Build history of the part. All positions in model axes, mm. Give positions to 0.01 mm unless a question says otherwise; leave off trailing zeros. Loops run counter-clockwise (first coordinate to the right, second up) from the corner with the lowest first, then second, coordinate; pieces in that order, holes last.
1) Wall check: line 1 (Z direction, x = 0, y = -228); line 2 (Y direction, x = 0.05, z = 16); line 3 (Z direction, x = 0.1, y = -166). Give the ranges that are in metal, low to high.
2) Band-saw the part on A-A on x = 0. List the corners of the cut face in (y, z).
3) Band-saw the part on B-B on y = -173. List the corners of the cut face in (x, z).
4) Flat gauge pin, fed straight in: P1, Ø6, axis at y = -182.5, z = 6.5, coming from the -X side. Where does the tip first touch, or does it go through?
```python
from build123d import *

# Parameters (mm, degrees)
NATIVE_HOLLOW_UTILITY_SWEEP_PROFILE_R = 0.18


with BuildPart() as part:
    # Native hollow utility sweep: sweep along a path in Illustrative smooth utility route
    with BuildLine(Plane(origin=(0, 0, 0), x_dir=(0, 0, -1), z_dir=(1, 0, 0))) as native_hollow_utility_sweep_path:
        Line((-15.85, 0), (-17.05, 0))
        ThreePointArc((-17.05, 0), (-17.262132034, -0.087867966), (-17.35, -0.3))
        Line((-17.35, -0.3), (-17.35, -17.32))
        ThreePointArc((-17.35, -17.32), (-15.642666611, -24.12589129), (-10.925, -29.32))
        ThreePointArc((-10.925, -29.32), (-6.207333389, -34.51410871), (-4.5, -41.32))
        Line((-4.5, -41.32), (-4.5, -277.32))
    # Native hollow utility sweep profile (on start of the path) → Native hollow utility sweep (sweep)
    with BuildSketch(Plane.XY.offset(15.85)):
        Circle(NATIVE_HOLLOW_UTILITY_SWEEP_PROFILE_R)
    sweep(path=native_hollow_utility_sweep_path.line)


solid = part.part
```
Findings below:
1. line 1: z = 4.32 to 4.68
1. line 2: y = -23.81 to -22.99, -0.17 to 0.17
1. line 3: z = 4.35 to 4.65
2. outline: (-277.32, 4.32) - (-41.32, 4.32) arc R14.6 ccw to (-29.17, 10.83) arc R14.24 cw to (-17.32, 17.17) - (-0.3, 17.17) arc R0.12 cw to (-0.18, 17.05) - (-0.18, 15.85) - (0.18, 15.85) - (0.18, 17.05) arc R0.48 ccw to (-0.3, 17.53) - (-17.32, 17.53) arc R14.6 ccw to (-29.47, 11.02) arc R14.24 cw to (-41.32, 4.68) - (-277.32, 4.68) - close
3. outline: circle Ø0.36 at (0, 4.5)
4. P1: stops at x = -0.18
